```python
from build123d import *

# Parameters (mm, degrees)
CUT_EXTRUDE1_DEPTH = 1.75


with BuildPart() as part:
    # Sketch2 → Revolve1 (revolve)
    with BuildSketch(Plane(origin=(0, 0, 0), x_dir=(0, 0, -1), z_dir=(1, 0, 0)), mode=Mode.PRIVATE) as revolve1_sk:
        with BuildLine():
            Line((-13.6, 0), (13.6, 0))
            Line((13.6, 0), (13.6, 1.44))
            Line((13.6, 1.44), (13.04, 2))
            Line((13.04, 2), (-11.4, 2))
            Line((-11.4, 2), (-11.4, 3.8))
            Line((-11.4, 3.8), (-11.73, 3.8))
            ThreePointArc((-11.73, 3.8), (-12.806499853, 3.047002626), (-13.6, 2))
            Line((-13.6, 2), (-13.6, 0))
        make_face()
    revolve(revolve1_sk.sketch.rotate(Axis((0, 0, 13.6), (0, 0, -1)), 90), axis=Axis((0, 0, 13.6), (0, 0, -1)))

    # Sketch3 → Cut-Extrude1 (cut)
    with BuildSketch(Plane.XY.offset(13.6)):
        Polygon((0, 1.443375673), (-1.25, 0.721687836), (-1.25, -0.721687836), (0, -1.443375673), (1.25, -0.721687836), (1.25, 0.721687836), align=None)
    extrude(amount=-CUT_EXTRUDE1_DEPTH, mode=Mode.SUBTRACT)

    # Cut-Extrude2 cone 1 section (through the dimple's axis) → Cut-Extrude2 (revolve, cut)
    with BuildSketch(Plane(origin=(0, 0, 13.6), x_dir=(0, -1, 0), z_dir=(1, 0, 0))):
        Polygon((0, 0), (1.443375673, 0), (0, 1.443375673), align=None)
    revolve(axis=Axis((0, 0, 13.6), (0, 0, -1)), mode=Mode.SUBTRACT)


solid = part.part
```
Geometry check sheet. Reference: the model listing, model coordinates, mm. A direction names the side the tool comes from. Coordinates: 2 decimals unless noted, no trailing zeros. Loops run counter-clockwise (first coordinate to the right, second up) from the corner with the lowest first, then second, coordinate; pieces in that order, holes last. Notation, with made-up numbers: (4.5, -10) - (41.5, -10) arc R9 cw to (41.5, -6) - close; hole circle Ø7 at (3.5, -4). An arc over 180 degrees is marked (long way). One line per item, written item: value. Start each with the question number.
(1) Mould release check, pull along Y, two halves, no side actions. Record for faces 1 (the flat face through (0, 0, -13.6)), 2 (the flat face through (-0.63, -1.08, 12.74)), 3 (the cylindrical face through (3.625, -1.141, 11.567)): released by +Y, released by -Y, zero draft, split by the parting line, or undercut.
(2) Material ranges on line 1 (Y direction, x = -0.25, z = 12.75); line 2 (Z direction, x = 0.5, y = 0); line 3 (X direction, y = -0.25, z = 8.25), recorded low to high. Write a range as [from, to].
(3) Depth check by flat-ended pin: P1, Ø3, axis at x = -0.5, z = 6, coming from the +Y side; P2, Ø3, axis at y = 1, z = 6.5, coming from the -X side; P3, Ø3, axis at x = 2.5, z = 7, coming from the -Y side. Enter the tip coordinate at first touch or a pass-through.
(4) Cross-section at C-C on x = 3. Enter the section's corners in (y, z).
(5) Tool access check on faces 4 (the flat face through (-2, 2, 11.4)), 5 (the flat face through (1.25, 0, 13)). Record the directions out of +Z, -Z, +X, -X, +Y, -Y that give a thin tool (end or side, any length) a straight path to the whole face; none if there is none.
(6) Cross-section at A-A on y = 0. Enter the section's corners in (x, z), plus the area to 3 significant figures.
(7) Cross-section at B-B on z = -7.75. Enter the section's corners in (x, y), plus the area to 3 significant figures.
Results below:
1. face 1: zero draft
1. face 2: undercut
1. face 3: split by the parting line
2. line 1: y = [-3.09, -1.3], [1.3, 3.09]
2. line 2: z = [-13.6, 11.85]
2. line 3: x = [-1.98, 1.98]
3. P1: stops at y = 2
3. P2: stops at x = -2
3. P3: stops at y = -1.73
4. outline: (-2.33, 11.4) - (2.33, 11.4) - (2.33, 11.73) arc R2.98 ccw to (-2.33, 11.73) - close
5. face 4: -Z
5. face 5: +Z
6. outline: (-3.8, 11.4) - (-2, 11.4) - (-2, -13.04) - (-1.44, -13.6) - (1.44, -13.6) - (2, -13.04) - (2, 11.4) - (3.8, 11.4) - (3.8, 11.73) arc R4.23 ccw to (2, 13.6) - (1.44, 13.6) - (1.25, 13.41) - (1.25, 11.85) - (-1.25, 11.85) - (-1.25, 13.41) - (-1.44, 13.6) - (-2, 13.6) arc R4.23 ccw to (-3.8, 11.73) - close
6. area: 109 mm2
7. outline: circle Ø4 at (0, 0)
7. area: 12.6 mm2
